```python
from build123d import *

# Parameters (mm, degrees)
BOSS_EXTRUDE2_DEPTH = 7
BOSS_EXTRUDE3_DEPTH = 15
FILLET1_R           = 2


with BuildPart() as part:
    # Sketch1 → Boss-Extrude2 (new body)
    with BuildSketch(Plane.XY):
        with BuildLine():
            Line((23.22459679983159, 11.838054320739976), (22.59461695676328, 29.0520343287084))
            Line((22.59461695676328, 29.052034328708398), (9.094616956763277, 29.052034328708398))
            Line((9.094616956763277, 29.052034328708398), (9.094616956763272, 2.8469015838410883))
            ThreePointArc((9.094616956763272, 2.846901583841089), (4.094616956763275, -2.153098416158908), (-0.9053830432367223, 2.8469015838410887))
            Line((-0.905383043236724, 2.846901583841089), (-0.9053830432367259, 24.399326740540857))
            Line((-0.9053830432367259, 24.399326740540857), (-9.372834944506629, 34.00764813303465))
            Line((-9.372834944506627, 34.00764813303465), (-19.338054555793107, 38.10430027910595))
            Line((-19.338054555793107, 38.10430027910595), (-27.64949584669558, 17.88648954074799))
            Line((-27.64949584669558, 17.886489540747988), (-39.54243331524863, 22.895355765149752))
            Line((-39.54243331524863, 22.895355765149752), (-39.54243331524862, -26.68595837588142))
            Line((-39.54243331524862, -26.68595837588142), (9.930508904802714, -18.62730077710855))
            ThreePointArc((9.93050890480271, -18.62730077710854), (21.888607340272777, -10.842166970276775), (26.528997575110665, 2.651209369657105))
            Line((26.528997575110658, 2.6512093696571015), (26.528997575110658, 6.583034036121315))
            Line((26.528997575110658, 6.583034036121315), (34.74430312273597, 6.583034036121314))
            Line((34.74430312273597, 6.583034036121314), (34.74430312273597, 11.35464156582886))
            Line((34.74430312273597, 11.35464156582886), (23.22459679983159, 11.838054320739976))
        make_face()
    extrude(amount=BOSS_EXTRUDE2_DEPTH)

    # Sketch1_7 → Boss-Extrude3 (add)
    with BuildSketch(Plane.XY):
        Polygon((-0.9053830432367259, 14.019993611037982), (-0.9053830432367259, 24.399326740540857), (-9.372834944506629, 34.00764813303465), (-19.338054555793107, 38.10430027910595), (-21.61937542853537, 32.55492418123779), (-11.654155817248892, 28.458272035166488), align=None)
        with BuildLine():
            ThreePointArc((20.523303512372856, 3.0772079508363284), (16.858734444980243, -7.523493754122956), (7.118615678125689, -13.085330635476565))
            Line((7.118615678125689, -13.085330635476566), (-39.542433315248616, -20.685958375881416))
            Line((-39.54243331524862, -20.685958375881416), (-39.54243331524862, -26.68595837588142))
            Line((-39.54243331524862, -26.68595837588142), (9.930508904802714, -18.62730077710855))
            ThreePointArc((9.93050890480271, -18.62730077710854), (21.888607340272777, -10.842166970276775), (26.528997575110665, 2.651209369657105))
            Line((26.528997575110658, 2.6512093696571015), (26.528997575110658, 6.583034036121315))
            Line((26.528997575110658, 6.583034036121315), (34.74430312273597, 6.583034036121314))
            Line((34.74430312273597, 6.583034036121314), (34.74430312273597, 11.35464156582886))
            Line((34.74430312273597, 11.35464156582886), (23.22459679983159, 11.838054320739976))
            Line((23.224596799831595, 11.838054320739976), (22.25718626662765, 10.122973627008314))
            Line((22.25718626662765, 10.122973627008314), (20.85012579434564, 5.080010210629205))
            Line((20.85012579434564, 5.080010210629205), (20.52330351237285, 3.0772079508363284))
        make_face()
        with BuildLine():
            ThreePointArc((-27.372162273437734, 3.6262968896540997), (-21.8978313295958, 10.087488754460773), (-26.30362524162322, 17.319658525787453))
            Line((-26.30362524162322, 17.319658525787453), (-39.54243331524863, 22.895355765149752))
            Line((-39.54243331524863, 22.895355765149752), (-39.54243331524863, -0.28742000905455))
            Line((-39.54243331524863, -0.28742000905455056), (-27.37216227343774, 3.626296889654118))
        make_face()
    extrude(amount=BOSS_EXTRUDE3_DEPTH)

    # Fillet1
    fillet1_edges = [part.edges().sort_by_distance(p)[0] for p in [
        (-21.61937542853537, 32.55492418123779, 11),
        (-0.9053830432367262, 14.019993611037982, 11),
        (-39.54243331524863, -0.2874200090545503, 11),
        (23.22459679983159, 11.838054320739976, 3.5),
        (34.74430312273597, 11.35464156582886, 7.5),
        (34.74430312273597, 6.583034036121314, 7.5),
        (-39.54243331524862, -26.68595837588142, 7.5),
        (-39.54243331524863, 22.895355765149752, 7.5),
        (-27.64949584669558, 17.886489540747988, 3.5),
        (-19.338054555793107, 38.10430027910595, 7.5),
        (-9.372834944506629, 34.00764813303465, 7.5),
        (-39.542433315248616, -20.685958375881416, 11),
    ]]
    fillet(fillet1_edges, radius=FILLET1_R)


solid = part.part
```
Part model, mm, in its own coordinate system. A direction names the side the tool comes from. Round coordinates to 2 decimals unless told otherwise and drop trailing zeros. Loops run counter-clockwise (first coordinate to the right, second up) from the corner with the lowest first, then second, coordinate; pieces in that order, holes last.
Item 1: Mould opens along X. For faces 4 (the face through (16, 29.052, 3)), 5 (the face through (-13.975, -22.521, 7.395)), 6 (the face through (-27.99, 18.655, 3.549)) say: +X half, -X half, draft (parallel to the pull), parting line (faces both ways), or undercut.
Item 2: 3-axis set-ups, long thin cutter, end or side, ignore diameter. For faces 1 (the face through (-32.218, 2.068, 10.944)), 2 (the face through (9.095, 16, 3)), 3 (the face through (-32.62, 19.98, 7.4)): which of +Z, -Z, +X, -X, +Y, -Y reach the whole face in a straight line?
Item 3: Cut at D-D, the plane z = 1.5. Give the cut face in (x, y), then the cut area to 3 significant figures.
Item 4: Cut at C-C, the plane x = 17.5. Give the cut face in (y, z).
Item 5: Cut at A-A, the plane z = 9.25. State how many separate pieces and enclosed holes the cut face has, then the cut area to 3 significant figures.
Item 6: Cut at B-B, the plane y = 27. Give the cut face in (x, z).
Item 7: Drop flat-ended pins along their axis: P1, Ø1.5, axis at x = 3.5, z = 9, coming from the -Y side; P2, Ø17, axis at x = -2.5, y = 14.5, coming from the +Z side; P3, Ø6, axis at x = -31.5, z = 12, coming from the +Y side; P4, Ø1.9, axis at x = 29.5, z = 5, coming from the -Y side. Give the stop position or say it passes through.
Item 8: Drill centre lines: line 1 (Z direction, x = -2.5, y = -9); line 2 (X direction, y = -1, z = 2.75); line 3 (X direction, y = 28, z = 5.5). Where is each one in solid material? Low to high.
A:
1. face 4: draft
1. face 5: +X half
1. face 6: undercut
2. face 1: +Z
2. face 2: +Z, -Z, +Y
2. face 3: +Z, +Y
3. outline: (-39.54, -24.33) arc R2 ccw to (-37.22, -26.31) - (9.93, -18.63) arc R21.94 ccw to (26.53, 2.65) - (26.53, 6.58) - (32.74, 6.58) arc R2 ccw to (34.74, 8.58) - (34.74, 9.44) arc R2 ccw to (32.83, 11.44) - (25.07, 11.76) arc R2 cw to (23.16, 13.69) - (22.59, 29.05) - (9.09, 29.05) - (9.09, 2.85) arc R5 cw to (-0.91, 2.85) - (-0.91, 24.4) - (-9.06, 33.66) arc R2 ccw to (-9.8, 34.19) - (-17.49, 37.34) arc R2 ccw to (-20.1, 36.25) - (-26.88, 19.75) arc R2 cw to (-29.51, 18.67) - (-36.77, 21.73) arc R2 ccw to (-39.54, 19.88) - close
3. area: 2,890 mm2
4. outline: (-15.09, 0) - (29.05, 0) - (29.05, 7) - (-6.7, 7) - (-6.7, 15) - (-15.09, 15) - close
5. separate pieces: 3
5. enclosed holes: 0
5. area: 953 mm2
6. outline: (-23.9, 0) - (-3.2, 0) - (-3.2, 15) - (-10.57, 15) - (-10.57, 7) - (-23.9, 7) - close; (9.09, 0) - (22.67, 0) - (22.67, 7) - (9.09, 7) - close
7. P1: stops at y = -19.8
7. P2: stops at z = 15
7. P3: stops at y = 20.77
7. P4: stops at y = 6.58
8. line 1: z = 0 to 7
8. line 2: x = -39.54 to 0.9, 7.29 to 26.22
8. line 3: x = -23.49 to -4.08, 9.09 to 22.63
